The listing builds one solid part. Answer for the finished solid, in the listing's coordinates (mm). Face numbers are marked on the shaded views. A direction names the side the tool comes from. Give positions to 0.01 mm unless a question says otherwise; leave off trailing zeros. Write each loop counter-clockwise with the first axis right and the second up, starting at its lowest first coordinate (ties: lowest second). Pieces come first, ordered by that corner, then holes. Notation, with made-up numbers: (25.5, 41) -> (43.5, 41) arc R17 cw to (43.5, 49) -> close; hole circle Ø10 at (20, -6). An arc over 180 degrees is marked (long way). One line per question, with ' | ' between items.
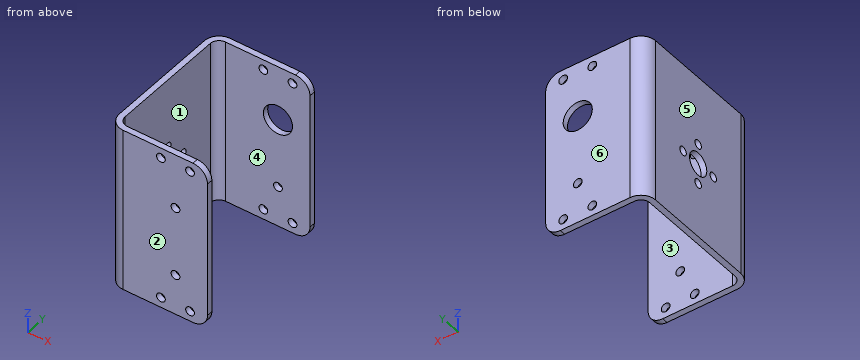
from build123d import *

# Parameters (mm, degrees)
EXTRUDE_1_DEPTH     = 57
SKETCH_2_R          = 1.5
CUT_EXTRUDE_1_DEPTH = 57
SKETCH_4_R          = 4
SKETCH_4_R_2        = 1.5
CUT_EXTRUDE_2_DEPTH = 57
FILLET_1_R          = 5
FILLET_2_R          = 3
FILLET_3_R          = 5
SKETCH_5_R          = 5
CUT_EXTRUDE_3_DEPTH = 26
SKETCH_6_R          = 1.5
CUT_EXTRUDE_4_DEPTH = 71


with BuildPart() as part:
    # 草图1 → 凸台-拉伸1 (new body)
    with BuildSketch(Plane.XY):
        Polygon((-17, -24.75), (17, -24.75), (17, -22.75), (-15, -22.75), (-15, 22.75), (17, 22.75), (17, 24.75), (-17, 24.75), align=None)
    extrude(amount=EXTRUDE_1_DEPTH)

    # 草图2 → 切除-拉伸1 (cut)
    with BuildSketch(Plane(origin=(0, 24.75, 0), x_dir=(1, 0, 0), z_dir=(0, 1, 0))):
        with Locations(Location((6, -14, 0), (0, 0, 270))):
            Circle(SKETCH_2_R)
        with Locations(Location((6, -38, 0), (0, 0, 270))):
            Circle(SKETCH_2_R)
    extrude(amount=-CUT_EXTRUDE_1_DEPTH, mode=Mode.SUBTRACT)

    # 草图4 → 切除-拉伸2 (cut)
    with BuildSketch(Plane.ZY.offset(17)):
        with Locations((26, 0)):
            Circle(SKETCH_4_R)
        with Locations((26, 7)):
            Circle(SKETCH_4_R_2)
        with Locations((33, 0)):
            Circle(SKETCH_4_R_2)
        with Locations((26, -7)):
            Circle(SKETCH_4_R_2)
        with Locations((19, 0)):
            Circle(SKETCH_4_R_2)
    extrude(amount=-CUT_EXTRUDE_2_DEPTH, mode=Mode.SUBTRACT)

    # 圆角1
    fillet_1_edges = [part.edges().sort_by_distance(p)[0] for p in [
        (-17, -24.75, 28.5),
        (-17, 24.75, 28.5),
    ]]
    fillet(fillet_1_edges, radius=FILLET_1_R)

    # 圆角2
    fillet_2_edges = [part.edges().sort_by_distance(p)[0] for p in [
        (-15, 22.75, 28.5),
        (-15, -22.75, 28.5),
    ]]
    fillet(fillet_2_edges, radius=FILLET_2_R)

    # 圆角3
    fillet_3_edges = [part.edges().sort_by_distance(p)[0] for p in [
        (17, 23.75, 0),
        (17, -23.75, 57),
        (17, 23.75, 57),
        (17, -23.75, 0),
    ]]
    fillet(fillet_3_edges, radius=FILLET_3_R)

    # 草图5 → 切除-拉伸3 (cut)
    with BuildSketch(Plane(origin=(0, 24.75, 0), x_dir=(1, 0, 0), z_dir=(0, 1, 0))):
        with Locations(Location((6, -38, 0), (0, 0, 270))):
            Circle(SKETCH_5_R)
    extrude(amount=-CUT_EXTRUDE_3_DEPTH, mode=Mode.SUBTRACT)

    # 草图6 → 切除-拉伸4 (cut)
    with BuildSketch(Plane.XZ.offset(24.75)):
        with Locations(Location((1, 53.5, 0), (0, 0, 270))):
            Circle(SKETCH_6_R)
        with Locations(Location((11, 53.5, 0), (0, 0, 270))):
            Circle(SKETCH_6_R)
        with Locations(Location((11, 3.5, 0), (0, 0, 270))):
            Circle(SKETCH_6_R)
        with Locations(Location((1, 3.5, 0), (0, 0, 270))):
            Circle(SKETCH_6_R)
    extrude(amount=-CUT_EXTRUDE_4_DEPTH, mode=Mode.SUBTRACT)


solid = part.part
Item 1: Find section A-A (z = 38). Write down the section's boundary in (x, y), then the cut area to 3 significant figures.
Answers below:
outline: (-17, -19.75) arc R5 ccw to (-12, -24.75) -> (4.5, -24.75) -> (4.5, -22.75) -> (-12, -22.75) arc R3 cw to (-15, -19.75) -> (-15, 19.75) arc R3 cw to (-12, 22.75) -> (1, 22.75) -> (1, 24.75) -> (-12, 24.75) arc R5 ccw to (-17, 19.75) -> close; (7.5, -24.75) -> (17, -24.75) -> (17, -22.75) -> (7.5, -22.75) -> close; (11, 22.75) -> (17, 22.75) -> (17, 24.75) -> (11, 24.75) -> close | area: 194 mm²
Item 2: Find section D-D (z = 26). Write down the section's boundary in (x, y), then the cut area to 3 significant figures.
Answers below:
outline: (-17, -19.75) arc R5 ccw to (-12, -24.75) -> (17, -24.75) -> (17, -22.75) -> (-12, -22.75) arc R3 cw to (-15, -19.75) -> (-15, -8.5) -> (-17, -8.5) -> close; (-17, -5.5) -> (-15, -5.5) -> (-15, -4) -> (-17, -4) -> close; (-17, 4) -> (-15, 4) -> (-15, 5.5) -> (-17, 5.5) -> close; (-17, 8.5) -> (-15, 8.5) -> (-15, 19.75) arc R3 cw to (-12, 22.75) -> (17, 22.75) -> (17, 24.75) -> (-12, 24.75) arc R5 ccw to (-17, 19.75) -> close | area: 192 mm²
Item 3: A tool of negligible diameter and unlimited length cuts with its end or side. For the marked faces 1 and 2, from which of +Z, -Z, +X, -X, +Y, -Y can it reach the whole face along a straight path? Write none if from no direction.
Answers below:
face 1: +Z, -Z, +X | face 2: +Z, -Z, +X, -X, -Y
Item 4: A flat-ended cylindrical pin translates along its axis: pin 1 (4 mm diameter, centred on y = -7, z = 26, fed in from +X). Find the tip coordinate at first contact, or state that the pin passes through.
Answers below:
pin 1: x = -15
Item 5: Determine the mould class of the marked faces 3, 4, 5 and 6 for opening direction Y: pulls with the +Y half, pulls with the -Y half, needs draft (parallel to the pull), parting line crosses it, or undercut.
Answers below:
face 3: undercut | face 4: undercut | face 5: needs draft | face 6: pulls with the +Y half
Item 6: Find section C-C (x = -4). Write down the section's boundary in (y, z), then the cut area to 3 significant figures.
Answers below:
outline: (-24.75, 0) -> (-22.75, 0) -> (-22.75, 57) -> (-24.75, 57) -> close; (22.75, 0) -> (24.75, 0) -> (24.75, 57) -> (22.75, 57) -> close | area: 228 mm²
Item 7: Find section B-B (y = 0). Write down the section's boundary in (x, z).
Answers below:
outline: (-17, 0) -> (-15, 0) -> (-15, 17.5) -> (-17, 17.5) -> close; (-17, 20.5) -> (-15, 20.5) -> (-15, 22) -> (-17, 22) -> close; (-17, 30) -> (-15, 30) -> (-15, 31.5) -> (-17, 31.5) -> close; (-17, 34.5) -> (-15, 34.5) -> (-15, 57) -> (-17, 57) -> close
Item 8: Consider line 1 (Y direction, x = -16, z = 26); line 2 (Y direction, x = -10.5, z = 49.5); line 3 (X direction, y = 23.4, z = 53.5). Determine where each line is inside the solid, lowest interval first. Write a range as [from, to].
Answers below:
line 1: [-22.75, -8.5], [-5.5, -4], [4, 5.5], [8.5, 22.75] | line 2: [-24.75, -22.75], [22.75, 24.75] | line 3: [-15.42, -0.5], [2.5, 9.5], [12.5, 16.77]
